```python
from build123d import *

# Parameters (mm, degrees)
F0_W          = 5.842
F0_H          = 12.7
F0_R          = 3.175
F2_DEPTH      = 3.175
F3_R          = 1.524
F4_DEPTH      = 7.62
F4_DEPTH_BACK = 1.27
F5_DEPTH      = 56.134


with BuildPart() as f1:
    # F0 (on Front) → F1 (revolve)
    with BuildSketch(Plane.XZ):
        Polygon((5.842, 12.7), (5.842, 0), (66.294, 0), (66.294, 12.7), (56.134, 12.7), (56.134, 10.16), (10.16, 10.16), (10.16, 12.7), align=None)
        with Locations((2.921, 6.35)):
            Rectangle(F0_W, F0_H)
    revolve(axis=Axis((33.147, 0, 0), (-1, 0, 0)))

    # F0 (on Front) → F2 (join, symmetric)
    with BuildSketch(Plane.XZ):
        with Locations((2.921, 6.35)):
            Rectangle(F0_W, F0_H)
        with BuildLine():
            Line((-0.9398, 0), (0, 0))
            Line((0, 0), (0, 12.7))
            Line((0, 12.7), (5.842, 12.7))
            Line((5.842, 12.7), (5.842, 15.24))
            Line((5.842, 15.24), (-0.508, 15.24))
            Line((-0.508, 15.24), (-10.8806298187, 3.8475430269))
            ThreePointArc((-10.8806298187, 3.8475430269), (-4.5919612295, 5.3297205562), (-0.9398, 0))
        make_face()
        with BuildLine():
            Line((5.842, 0), (0, 0))
            Line((0, 0), (-0.9398, 0))
            ThreePointArc((-0.9398, 0), (-3.1957909266, -4.5493385486), (-8.1826630726, -5.5069827884))
            Line((-8.1826630726, -5.5069827884), (5.842, -9.398))
            Line((5.842, -9.398), (5.842, 0))
        make_face()
        with BuildLine():
            ThreePointArc((-8.1826630726, -5.5069827884), (-3.1957909266, -4.5493385486), (-0.9398, 0))
            ThreePointArc((-0.9398, 0), (-4.5919612295, 5.3297205562), (-10.8806298187, 3.8475430269))
            ThreePointArc((-10.8806298187, 3.8475430269), (-12.1459778134, -1.5837270034), (-8.1826630726, -5.5069827884))
        make_face()
        with Locations((-6.6548, 0)):
            Circle(F0_R, mode=Mode.SUBTRACT)
    extrude(amount=F2_DEPTH, both=True)

    # F3 (on face) → F4 (join, two sides)
    with BuildSketch(Plane.YZ.offset(66.294)) as f4_sk:
        with BuildLine():
            ThreePointArc((-5.08, 0), (0, -5.08), (5.08, 0))
            ThreePointArc((5.08, 0), (0, 5.08), (-5.08, 0))
        make_face()
        Circle(F3_R, mode=Mode.SUBTRACT)
        with BuildLine():
            ThreePointArc((-5.08, 0), (0, 5.08), (5.08, 0))
            Line((5.08, 0), (5.08, 15.24))
            Line((5.08, 15.24), (-5.08, 15.24))
            Line((-5.08, 15.24), (-5.08, 0))
        make_face()
    extrude(amount=F4_DEPTH)
    extrude(f4_sk.sketch, amount=-F4_DEPTH_BACK)

    # F5 (add, through all): a face of the model
    f5_faces = [f1.faces().sort_by_distance(p)[0] for p in [
        (66.294, 0, 0),
    ]]
    extrude(f5_faces, amount=-F5_DEPTH)


solid = f1.part
```
Part model, mm, in its own coordinate system. A direction names the side the tool comes from. Round coordinates to 2 decimals unless told otherwise and drop trailing zeros. Loops run counter-clockwise (first coordinate to the right, second up) from the corner with the lowest first, then second, coordinate; pieces in that order, holes last. Notation, with made-up numbers: (-21.5, 67.25) -> (-0.5, 67.25) arc R25 cw to (-0.5, 97.25) -> close; hole circle Ø9 at (28, 57). An arc over 180 degrees is marked (long way). Use a Markdown table: item, result.
1) Cut at C-C, the plane x = 61.5. List the corners of the cut face in (y, z).
The answers:
| item | result |
|---|---|
| outline | circle Ø25.4 at (0, 0) |
2) Cut at A-A, the plane y = 0. List the corners of the cut face in (x, z) (3 decimals), and give its area (3 significant figures).
The answers:
| item | result |
|---|---|
| outline | (-10.881, 3.848) arc R5.715 ccw to (-8.183, -5.507) -> (0, -7.777) -> (0, -12.7) -> (10.16, -12.7) -> (10.16, -10.16) -> (56.134, -10.16) -> (56.134, -12.7) -> (66.294, -12.7) -> (66.294, -5.08) -> (73.914, -5.08) -> (73.914, -1.524) -> (66.294, -1.524) -> (66.294, 1.524) -> (73.914, 1.524) -> (73.914, 15.24) -> (65.024, 15.24) -> (65.024, 12.7) -> (56.134, 12.7) -> (56.134, 10.16) -> (10.16, 10.16) -> (10.16, 12.7) -> (5.842, 12.7) -> (5.842, 15.24) -> (-0.508, 15.24) -> close; hole circle Ø6.35 at (-6.655, 0) |
| area | 1,750 mm2 |
3) Cut at B-B, the plane z = 13.5. List the corners of the cut face in (x, y) (3 decimals), and give its area (3 significant figures).
The answers:
| item | result |
|---|---|
| outline | (-2.092, -3.175) -> (5.842, -3.175) -> (5.842, 3.175) -> (-2.092, 3.175) -> close; (65.024, -5.08) -> (73.914, -5.08) -> (73.914, 5.08) -> (65.024, 5.08) -> close |
| area | 141 mm2 |
4) Cut at D-D, the plane y = 6. List the corners of the cut face in (x, z).
The answers:
| item | result |
|---|---|
| outline | (0, -11.19) -> (10.16, -11.19) -> (10.16, -8.2) -> (56.13, -8.2) -> (56.13, -11.19) -> (66.29, -11.19) -> (66.29, 11.19) -> (56.13, 11.19) -> (56.13, 8.2) -> (10.16, 8.2) -> (10.16, 11.19) -> (0, 11.19) -> close |
5) Drop flat-ended pins along their axis: pin 1 Ø0.9 at (y, z) = (0.5, -0.5) entering from +X; pin 2 Ø12 at (x, y) = (9.5, -10) entering from +Z; pin 3 Ø1.1 at (y, z) = (-2, 13) entering from -X. Give the stop position or say it passes through.
The answers:
| item | result |
|---|---|
| pin 1 | stops at x = 66.29 |
| pin 2 | stops at z = 12.05 |
| pin 3 | stops at x = -3.05 |
6) Pull direction X, two halves, no side cores. Call faces 1 (the flat face through (5.842, 0, 14)), 2 (the flat face through (-3, -3.175, 4)), 3 (the cylindrical face through (32.825, 10.074, -1.323)), 4 (the flat face through (73.914, 0, 5)): pulls with the +X half, pulls with the -X half, needs draft (parallel to the pull), parting line crosses it, or undercut.
The answers:
| item | result |
|---|---|
| face 1 | undercut |
| face 2 | needs draft |
| face 3 | undercut |
| face 4 | pulls with the +X half |
7) Probe line 1 (X direction, y = 9, z = 6.75); line 2 (X direction, y = -4.25, z = 9.5); line 3 (X direction, y = 3.75, z = 8.75). List the from-to ranges inside material, lowest first. Write a range as [from, to].
The answers:
| item | result |
|---|---|
| line 1 | x = [0, 10.16], [56.13, 66.29] |
| line 2 | x = [0, 10.16], [56.13, 73.91] |
| line 3 | x = [0, 73.91] |
8) Tool access for faces 5 (the flat face through (10.16, 9, 6)), 6 (the flat face through (66.294, 0, 0)), 7 (the cylindrical face through (70.05, -0.11, -5.08)), 8 (the flat face through (0, -5, 0)): list every direction of +Z, -Z, +X, -X, +Y, -Y with a clear straight run to the whole face (end or side of a thin tool).
The answers:
| item | result |
|---|---|
| face 5 | none |
| face 6 | +X |
| face 7 | -Z, +X |
| face 8 | -Z, -X |
